Here's how the part is built. I have some questions about the finished solid (model axes, mm). A direction names the side the tool comes from. Round coordinates to 2 decimals unless told otherwise and drop trailing zeros. Write each loop counter-clockwise with the first axis right and the second up, starting at its lowest first coordinate (ties: lowest second). Pieces come first, ordered by that corner, then holes. Notation, with made-up numbers: (6.25, -18.5) -> (35.25, -18.5) arc R17 cw to (35.25, -9.5) -> close; hole circle Ø11 at (-5.75, 6.25). An arc over 180 degrees is marked (long way). Answer in a Markdown table with one row per item.
from build123d import *

# Parameters (mm, degrees)
BOSS_EXTRUDE1_DEPTH      = 3.81
BOSS_EXTRUDE1_DEPTH_BACK = 19.05
SKETCH1_R                = 7.9375
SKETCH2_R                = 6.35
BOSS_EXTRUDE2_DEPTH      = 31.75
CHAMFER1_SIZE            = 1.5875
CHAMFER2_SIZE            = 0.79375
SKETCH3_W                = 3.048
SKETCH3_H                = 1.524
CUT_EXTRUDE1_DEPTH       = 25.4


with BuildPart() as part:
    # Sketch1 → Boss-Extrude1 (new, two sides: drawn at the far end of the back side and taken through both)
    with BuildSketch(Plane.XY.offset(-BOSS_EXTRUDE1_DEPTH_BACK)):
        Circle(SKETCH1_R)
    extrude(amount=BOSS_EXTRUDE1_DEPTH + BOSS_EXTRUDE1_DEPTH_BACK)

    # Sketch2 → Boss-Extrude2 (add)
    with BuildSketch(Plane.XY.offset(3.81)):
        Circle(SKETCH2_R)
    extrude(amount=BOSS_EXTRUDE2_DEPTH)

    # Chamfer1
    chamfer1_edges = [part.edges().sort_by_distance(p)[0] for p in [
        (-7.9375, 0, 3.81),
    ]]
    chamfer(chamfer1_edges, length=CHAMFER1_SIZE - 0.0001)  # a hair under: the kernel refuses the full size

    # Chamfer2
    chamfer2_edges = [part.edges().sort_by_distance(p)[0] for p in [
        (-6.35, 0, 35.56),
    ]]
    chamfer(chamfer2_edges, length=CHAMFER2_SIZE)

    # Sketch3 → Cut-Extrude1 (cut)
    with BuildSketch(Plane.XY.offset(35.56)):
        with Locations((0, 5.588)):
            Rectangle(SKETCH3_W, SKETCH3_H)
    extrude(amount=-CUT_EXTRUDE1_DEPTH, mode=Mode.SUBTRACT)


solid = part.part
1) Which directions (+Z, -Z, +X, -X, +Y, -Y) give clear straight access to the entire face, cutting with the end or side of a thin tool? Please do faces 1 (the face through (1.524, 5, 23)), 2 (the face through (-1.38, -6.2, 19.07)), 3 (the face through (0, 0, 35.56)).
Response:
| item | result |
|---|---|
| face 1 | +Z, +Y |
| face 2 | +Z |
| face 3 | +Z, +X, -X, +Y, -Y |
2) I want a section at C-C, the plane z = -5.5. List the corners of the cut face in (x, y) for me (1 decimal).
Response:
| item | result |
|---|---|
| outline | circle Ø15.9 at (0, 0) |
3) I need wall thicknesses on line 1 (X direction, y = 5, z = 31); line 2 (X direction, y = 5.5, z = 32); line 3 (Y direction, x = 4, z = -5). Which ranges of each line are inside material? Lowest first, please. Write a range as [from, to].
Response:
| item | result |
|---|---|
| line 1 | x = [-3.91, -1.52], [1.52, 3.91] |
| line 2 | x = [-3.17, -1.52], [1.52, 3.17] |
| line 3 | y = [-6.86, 6.86] |
4) We'd pull the mould along X, two halves only. Please class faces 4 (the face through (-1.72, -7.75, -8.56)), 5 (the face through (0, 4.826, 23)), 6 (the face through (0, 0, -19.05)): +X half, -X half, draft (parallel to the pull), parting line (faces both ways), or undercut.
Response:
| item | result |
|---|---|
| face 4 | parting line |
| face 5 | undercut |
| face 6 | draft |
5) I want a section at D-D, the plane z = 19. List the corners of the cut face in (x, y) for me, and give its area (3 significant figures).
Response:
| item | result |
|---|---|
| outline | (-1.52, 4.83) -> (-1.52, 6.16) arc R6.35 ccw (long way) to (1.52, 6.16) -> (1.52, 4.83) -> close |
| area | 122 mm^2 |
6) For pin 1 (1.5 mm diameter, centred on x = 0.5, z = 23, fed in from +Y); pin 2 (3 mm diameter, centred on x = 4, z = 11.5, fed in from +Y); pin 3 (0.7 mm diameter, centred on y = 5.5, z = 27.5, fed in from -X); pin 4 (6 mm diameter, centred on x = -2.5, y = 5, fed in from +Z), each with a flat end and sliding along its axis, tell me the tip position at first contact or that it passes through.
Response:
| item | result |
|---|---|
| pin 1 | stops at y = 4.83 |
| pin 2 | stops at y = 5.84 |
| pin 3 | stops at x = -3.71 |
| pin 4 | stops at z = 35.56 |
